Autodesk Inventor part; units mm, degrees
ref_plane "YZ Plane" through (0, 0, 0) normal (1, 0, 0) x (0, 1, 0)
ref_plane "XZ Plane" through (0, 0, 0) normal (0, 1, 0) x (-1, 0, 0)
ref_plane "XY Plane" through (0, 0, 0) normal (0, 0, 1) x (1, 0, 0)
sketch "Sketch1" plane through (0, 0, 0) normal (0, 0, 1) x (1, 0, 0)
  line L0 (-2, -12.5) -> (2, -12.5)
  line L1 (2, -12.5) -> (2, 12.5)
  line L2 (2, 12.5) -> (-2, 12.5)
  line L3 (-2, 12.5) -> (-2, -12.5)
  line L4 (-2, -12.5) -> (2, 12.5) construction
  line L5 (2, -12.5) -> (-2, 12.5) construction
  line L6 (-4.5, -15) -> (4.5, -15)
  line L7 (4.5, -15) -> (4.5, 15)
  line L8 (4.5, 15) -> (-4.5, 15)
  line L9 (-4.5, 15) -> (-4.5, -15)
  line L10 (-4.5, -15) -> (4.5, 15) construction
  line L11 (4.5, -15) -> (-4.5, 15) construction
  point P0 (0, 0)
  dimension "d0" = 4
  dimension "d1" = 25
  dimension "d2" = 9
  dimension "d3" = 30
extrude "Extrusion1" add sketch "Sketch1" along normal blind 13
fillet "Fillet1" radius 3 4 edges at (-4.5, 15, 6.5) (4.5, 15, 6.5) (4.5, -15, 6.5) (-4.5, -15, 6.5)
fillet "Fillet2" radius 0.5 16 edges at (-3.6213, 14.1213, 13) (-4.5, 0, 13) (-3.6213, -14.1213, 13) (0, -15, 13) (3.6213, -14.1213, 13) (4.5, 0, 13) (3.6213, 14.1213, 13) (0, 15, 13) (-3.6213, 14.1213, 0) (-4.5, 0, 0) (-3.6213, -14.1213, 0) (0, -15, 0) (3.6213, -14.1213, 0) (4.5, 0, 0) (3.6213, 14.1213, 0) (0, 15, 0)
properties part number "copper-wire"
CAD build for the part. Positions are in the model's coordinates, mm. A direction names the side the tool comes from. Round coordinates to 2 decimals unless told otherwise and drop trailing zeros. Order: outer loops, then holes, each group sorted by start corner. A loop starts at its lowest first (then second) coordinate and runs counter-clockwise, first axis right, second up.
Item 1: Saw through at A-A on z = 4. Write the cut outline in (x, y), then the cut area to 3 significant figures.
Item 2: Saw through at B-B on y = -5. Write the cut outline in (x, z).
Item 3: Mould opens along X. For faces 3 (the face through (-3.64, -14.1, 6.58)), 4 (the face through (4.5, 0, 6)), 5 (the face through (2, 0, 6)) say: pulls with the +X half, pulls with the -X half, needs draft (parallel to the pull), parting line crosses it, or undercut.
Item 4: Saw through at C-C on x = 0.25. Write the cut outline in (y, z), then the cut area to 3 significant figures.
Item 5: Tool access for faces 1 (the face through (-2, 0, 6)), 2 (the face through (0, -15, 6)): list every direction of +Z, -Z, +X, -X, +Y, -Y with a clear straight run to the whole face (end or side of a thin tool).
Item 6: Probe line 1 along X through (y, z) = (6, 1.5); line 2 along Y through (x, z) = (0.5, 6.25); line 3 along Y through (x, z) = (-1.25, 12.75). List the from-to ranges inside material, lowest first.
Reported:
1. outline: (-4.5, -12) arc R3 ccw to (-1.5, -15) - (1.5, -15) arc R3 ccw to (4.5, -12) - (4.5, 12) arc R3 ccw to (1.5, 15) - (-1.5, 15) arc R3 ccw to (-4.5, 12) - close; hole (-2, -12.5) - (2, -12.5) - (2, 12.5) - (-2, 12.5) - close
1. area: 162 mm2
2. outline: (-4.5, 0.5) arc R0.5 ccw to (-4, 0) - (-2, 0) - (-2, 13) - (-4, 13) arc R0.5 ccw to (-4.5, 12.5) - close; (2, 0) - (4, 0) arc R0.5 ccw to (4.5, 0.5) - (4.5, 12.5) arc R0.5 ccw to (4, 13) - (2, 13) - close
3. face 3: pulls with the -X half
3. face 4: pulls with the +X half
3. face 5: undercut
4. outline: (-15, 0.5) arc R0.5 ccw to (-14.5, 0) - (-12.5, 0) - (-12.5, 13) - (-14.5, 13) arc R0.5 ccw to (-15, 12.5) - close; (12.5, 0) - (14.5, 0) arc R0.5 ccw to (15, 0.5) - (15, 12.5) arc R0.5 ccw to (14.5, 13) - (12.5, 13) - close
4. area: 64.8 mm2
5. face 1: +Z, -Z
5. face 2: +Z, -Z, +X, -X, -Y
6. line 1: x = -4.5 to -2, 2 to 4.5
6. line 2: y = -15 to -12.5, 12.5 to 15
6. line 3: y = -14.93 to -12.5, 12.5 to 14.93
